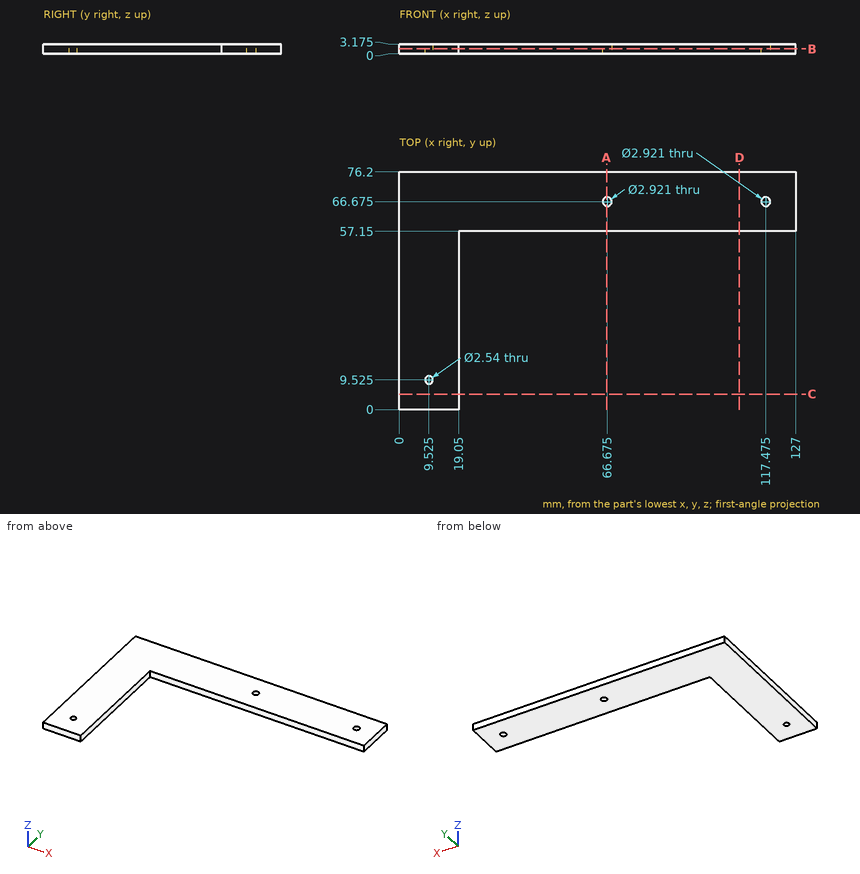
Can you work these out from the drawing? Everything is in mm from the part's minimum corner. Give positions to 0.01 mm unless a question says otherwise; leave off trailing zeros. Write each loop counter-clockwise with the first axis right and the second up, starting at its lowest first coordinate (ties: lowest second). Pieces come first, ordered by that corner, then holes. Notation, with made-up numbers: (14.25, 10.5) -> (62.25, 10.5) arc R20 cw to (62.25, 21.5) -> close; hole circle Ø5 at (-31.75, 9). An arc over 180 degrees is marked (long way). Write each question's results on one line, items separated by ' | '.
Item 1: Suppose I cut it at C-C on y = 5. Write out the boundary of the cut face in (x, z) (3 decimals), plus the area to 3 significant figures.
Output:
outline: (0, 0) -> (19.05, 0) -> (19.05, 3.175) -> (0, 3.175) -> close | area: 60.5 mm^2
Item 2: If I drill on L1, parallel to X at y = 67, z = 1.7; L2, parallel to X at y = 6, z = 3.05; L3, parallel to Y at x = 114, z = 1.45, over which ranges is the centre line in solid material (lowest first)?
Output:
L1: x = 0 to 65.25, 68.1 to 116.05, 118.9 to 127 | L2: x = 0 to 19.05 | L3: y = 57.15 to 76.2
Item 3: Suppose I cut it at A-A on x = 66.5. Write out the boundary of the cut face in (y, z) (3 decimals), plus the area to 3 significant figures.
Output:
outline: (57.15, 0) -> (65.225, 0) -> (65.225, 3.175) -> (57.15, 3.175) -> close; (68.125, 0) -> (76.2, 0) -> (76.2, 3.175) -> (68.125, 3.175) -> close | area: 51.3 mm^2
Item 4: Suppose I cut it at D-D on x = 109. Write out the boundary of the cut face in (y, z) (3 decimals), plus the area to 3 significant figures.
Output:
outline: (57.15, 0) -> (76.2, 0) -> (76.2, 3.175) -> (57.15, 3.175) -> close | area: 60.5 mm^2
Item 5: For pin 1 Ø1 at (y, z) = (17.5, 2.5) entering from +X, with a flat end and sliding along its axis, tell me the tip position at first contact or that it passes through.
Output:
pin 1: stops at x = 19.05
Item 6: Suppose I cut it at B-B on z = 1.6. Give the number of separate pieces and of enclosed holes in the cut face, plus the area to 3 significant figures.
Output:
separate pieces: 1 | enclosed holes: 3 | area: 3,490 mm^2
